```python
from build123d import *

# Parameters (mm, degrees)
PAD_DEPTH       = 30
THICKNESS_T     = 1
SKETCH001_R     = 0.75
SKETCH001_W     = 12.5
SKETCH001_H     = 23
POCKET_DEPTH    = 5
SKETCH002_R     = 0.75
POCKET001_DEPTH = 1
FILLET001_R     = 0.5
FILLET_R        = 0.5


with BuildPart() as part:
    # Sketch → Pad (new body)
    with BuildSketch(Plane.XY):
        Polygon((-15, 120), (-15, 0), (0, -30), (15, 0), (15, 120), align=None)
    extrude(amount=PAD_DEPTH)

    # Thickness
    thickness_openings = [part.faces().sort_by_distance(p)[0] for p in [
        (0, 52.222222, 30),
    ]]
    offset(amount=THICKNESS_T, openings=thickness_openings)

    # Sketch001 (on Face6 of Thickness) → Pocket (cut)
    with BuildSketch(Plane.XY):
        with Locations((0, 19)):
            Circle(SKETCH001_R)
        with Locations((0, -8)):
            Circle(SKETCH001_R)
        with Locations((0, 5.5)):
            Rectangle(SKETCH001_W, SKETCH001_H)
    extrude(amount=-POCKET_DEPTH, mode=Mode.SUBTRACT)

    # Sketch002 (on Face15 of Pocket) → Pocket001 (cut)
    with BuildSketch(Plane(origin=(0, 121, 0), x_dir=(-1, 0, 0), z_dir=(0, 1, 0))):
        with Locations((-8, 15)):
            Circle(SKETCH002_R)
        with Locations((8, 15)):
            Circle(SKETCH002_R)
    extrude(amount=-POCKET001_DEPTH, mode=Mode.SUBTRACT)

    # Fillet001
    fillet001_edges = [part.edges().sort_by_distance(p)[0] for p in [
        (0, -30, 15),
        (15, 0, 15),
        (-15, 0, 15),
        (-15, 120, 15),
        (15, 120, 15),
    ]]
    fillet(fillet001_edges, radius=FILLET001_R)

    # Fillet
    fillet_edges = [part.edges().sort_by_distance(p)[0] for p in [
        (7.697214, -14.605573, 0),
        (0, -29.381966, 0),
        (-7.697214, -14.605573, 0),
        (15, 59.809017, 0),
        (14.986624, 0.003158, 0),
        (-14.986624, 0.003158, 0),
        (-15, 59.809017, 0),
        (0, 120, 0),
        (14.853553, 119.853553, 0),
        (-14.853553, 119.853553, 0),
    ]]
    fillet(fillet_edges, radius=FILLET_R)


solid = part.part
```
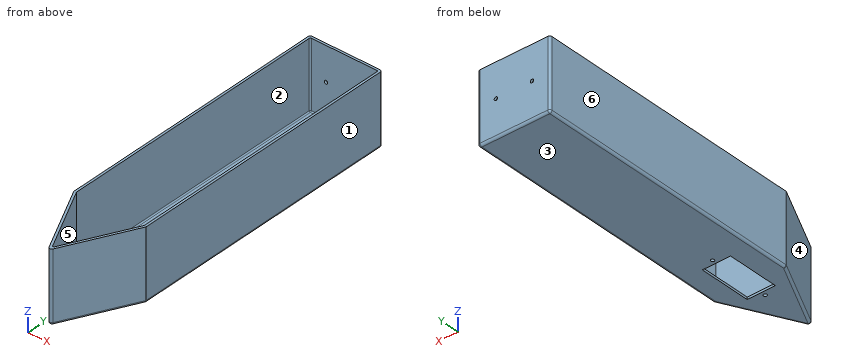
Can you work these out from the model? Positions are in its coordinate system, mm. Face numbers are marked on the shaded views. A direction names the side the tool comes from. Round coordinates to 2 decimals unless told otherwise and drop trailing zeros. Loops run counter-clockwise (first coordinate to the right, second up) from the corner with the lowest first, then second, coordinate; pieces in that order, holes last. Notation, with made-up numbers: M 88,62.5 L 101,62.5 A17 ccw 101,75.5 Z; hole C -19.75,-17.5 d9. An arc over 180 degrees is marked long. Answer as a JSON object with one key per item and string values. Group by question number.
Q1. Please list where these lines run through material, in increasing order: L1, parallel to X at y = 52, z = 5; L2, parallel to Y at x = 0, z = -0.8; L3, parallel to Y at x = 0, z = -0.55.
Q2. We'd pull the mould along X, two halves only. Please class the marked faces 1, 2, 3 and 4: +X half, -X half, draft (parallel to the pull), parting line (faces both ways), or undercut.
Q3. Imagine slicing it at A-A, the plane z = 10. Please give me the cut outline in (x, y), then the cut area to 3 significant figures.
Q4. Will these pins go through, and if not, where does the flat tip stop? pin 1 (14.5 mm diameter, centred on x = 1.5, y = 65, fed in from +Z); pin 2 (12 mm diameter, centred on x = 11.5, z = 24, fed in from -Y); pin 3 (0.9 mm diameter, centred on x = 8, z = 15, fed in from +Y); pin 4 (1.4 mm diameter, centred on x = 0, y = 19, fed in from -Z).
Q5. Imagine slicing it at B-B, the plane y = 55. Please give me the cut outline in (x, z), then the cut area to 3 significant figures.
Q6. On a 3-axis mill with a long thin cutter (end or side, diameter ignored), from which of +Z, -Z, +X, -X, +Y, -Y can I reach the whole of each face in a straight line? I mean the marked faces 5 and 6. Say none if no direction works.
Findings:
{
 "1": {"L1": "x = -16 to -15, 15 to 16", "L2": "y = -30.6 to -8.75, -7.25 to -6, 17 to 18.25, 19.75 to 120.6", "L3": "y = -30.84 to -8.75, -7.25 to -6, 17 to 18.25, 19.75 to 120.84"},
 "2": {"face 1": "+X half", "face 2": "undercut", "face 3": "draft", "face 4": "-X half"},
 "3": {"outline": "M -16,0 A1 ccw -15.89,-0.45 L -0.89,-30.45 A1 ccw 0.89,-30.45 L 15.89,-0.45 A1 ccw 16,0 L 16,120 A1 ccw 15,121 L -15,121 A1 ccw -16,120 Z; hole M -15,0.12 A0.5 ccw -14.95,-0.11 L -0.45,-29.11 A0.5 ccw 0.45,-29.11 L 14.95,-0.11 A0.5 ccw 15,0.12 L 15,119.5 A0.5 ccw 14.5,120 L -14.5,120 A0.5 ccw -15,119.5 Z", "area": "341 mm2"},
 "4": {"pin 1": "stops at z = 0", "pin 2": "stops at y = -21.24", "pin 3": "stops at y = -13.1", "pin 4": "passes through"},
 "5": {"outline": "M -16,0 A1 ccw -15,-1 L 15,-1 A1 ccw 16,0 L 16,30 L 15,30 L 15,0.5 A0.5 cw 14.5,0 L -14.5,0 A0.5 cw -15,0.5 L -15,30 L -16,30 Z", "area": "91.7 mm2"},
 "6": {"face 5": "+Z", "face 6": "+Z, -Z, -X, +Y, -Y"}
}
